Here's how the part is built. I have some questions about the finished solid (model axes, mm). Face numbers are marked on the shaded views. A direction names the side the tool comes from. Coordinates: 2 decimals unless noted, no trailing zeros. Loops run counter-clockwise (first coordinate to the right, second up) from the corner with the lowest first, then second, coordinate; pieces in that order, holes last.
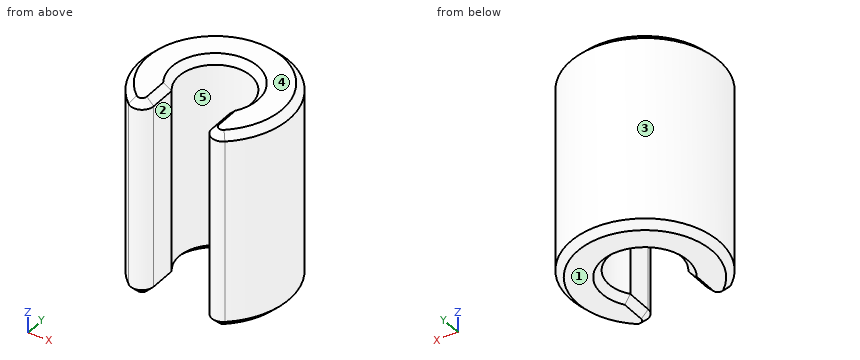
```python
from build123d import *

# Parameters (mm, degrees)
F1_DEPTH = 17
F2_R     = 1
F3_SIZE  = 0.6


with BuildPart() as f1:
    # F0 (on Top) → F1 (new body)
    with BuildSketch(Plane.XY):
        with BuildLine():
            ThreePointArc((-2.5, -1.83303), (0, 3.1), (2.5, -1.83303))
            Line((2.5, -1.83303), (2.5, -5.891519))
            ThreePointArc((2.5, -5.891519), (0, 6.4), (-2.5, -5.891519))
            Line((-2.5, -5.891519), (-2.5, -1.83303))
        make_face()
    extrude(amount=F1_DEPTH)

    # F2
    f2_edges = [f1.edges().sort_by_distance(p)[0] for p in [
        (-2.5, -5.891519, 8.5),
        (2.5, -5.891519, 8.5),
    ]]
    fillet(f2_edges, radius=F2_R)

    # F3
    f3_edges = [f1.edges().sort_by_distance(p)[0] for p in [
        (-2.5, -2.972604, 17),
        (-3.080565, -5.019962, 17),
        (0, 3.1, 17),
        (0, 6.4, 17),
        (2.5, -2.972604, 17),
        (3.080565, -5.019962, 17),
        (-2.5, -2.972604, 0),
        (-3.080565, -5.019962, 0),
        (0, 3.1, 0),
        (0, 6.4, 0),
        (2.5, -2.972604, 0),
        (3.080565, -5.019962, 0),
    ]]
    chamfer(f3_edges, length=F3_SIZE)


solid = f1.part
```
1. I want a section at A-A (y = 0). Please give me the cut outline in (x, z).
2. On a 3-axis mill with a long thin cutter (end or side, diameter ignored), from which of +Z, -Z, +X, -X, +Y, -Y can I reach the whole of each face in a straight line? I mean the marked faces 1 and 2. Say none if no direction works.
3. For pin 1 (6 mm diameter, centred on y = 4, z = 2.5, fed in from -X); pin 2 (6 mm diameter, centred on y = 4, z = 14.5, fed in from +X); pin 3 (5 mm diameter, centred on x = 2, z = 11.5, fed in from -Y); pin 4 (2.5 mm diameter, centred on y = -3.5, z = 9.5, fed in from +X), each with a flat end and sliding along its axis, tell me the tip position at first contact or that it passes through.
4. I want a section at C-C (z = 9). Please give me the cut outline in (x, y), then the cut area to 3 significant figures.
5. We'd pull the mould along X, two halves only. Please class the marked faces 3, 4 and 5: +X half, -X half, draft (parallel to the pull), parting line (faces both ways), or undercut.
6. I want a section at B-B (x = 0). Please give me the cut outline in (y, z), then the cut area to 3 significant figures.
7. I need wall thicknesses on line 1 along X through (y, z) = (0, 8.5); line 2 along Y through (x, z) = (0, 6.25); line 3 along X through (y, z) = (1.75, 4.75). Which ranges of each line are inside material? Lowest first, please.
Response values:
1. outline: (-6.4, 0.6) - (-5.8, 0) - (-3.7, 0) - (-3.1, 0.6) - (-3.1, 16.4) - (-3.7, 17) - (-5.8, 17) - (-6.4, 16.4) - close; (3.1, 0.6) - (3.7, 0) - (5.8, 0) - (6.4, 0.6) - (6.4, 16.4) - (5.8, 17) - (3.7, 17) - (3.1, 16.4) - close
2. face 1: -Z, +X, -X, +Y, -Y
2. face 2: +Z, -Z, -Y
3. pin 1: stops at x = -6.32
3. pin 2: stops at x = 6.32
3. pin 3: stops at y = -5.11
3. pin 4: stops at x = 5.99
4. outline: (-4.15, -4.87) arc R1 ccw to (-2.5, -4.11) - (-2.5, -1.83) arc R3.1 cw (long way) to (2.5, -1.83) - (2.5, -4.11) arc R1 ccw to (4.15, -4.87) arc R6.4 ccw (long way) to start
4. area: 79.3 mm2
5. face 3: parting line
5. face 4: draft
5. face 5: undercut
6. outline: (3.1, 0.6) - (3.7, 0) - (5.8, 0) - (6.4, 0.6) - (6.4, 16.4) - (5.8, 17) - (3.7, 17) - (3.1, 16.4) - close
6. area: 55.4 mm2
7. line 1: x = -6.4 to -3.1, 3.1 to 6.4
7. line 2: y = 3.1 to 6.4
7. line 3: x = -6.16 to -2.56, 2.56 to 6.16
